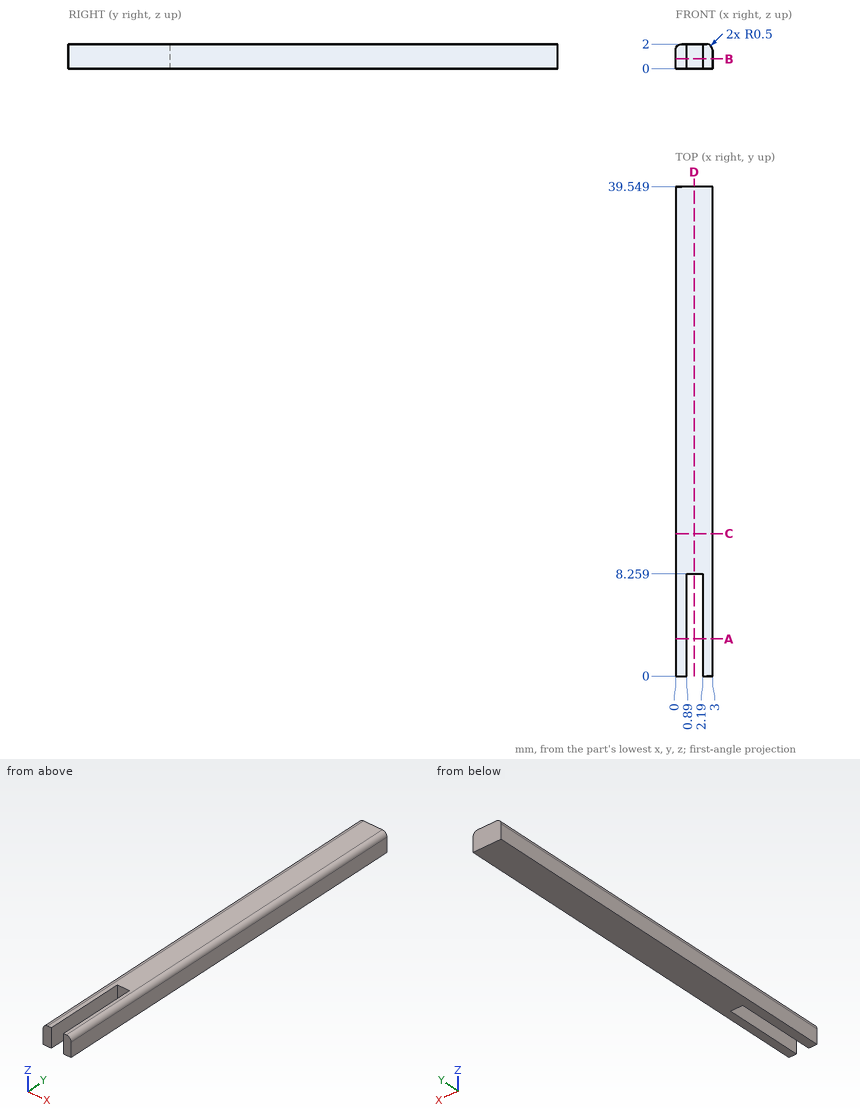
Check sheet for the drawn part. Datum: minimum x, y, z corner. Units: mm. Give positions to 0.01 mm unless a question says otherwise; leave off trailing zeros. Order: outer loops, then holes, each group sorted by start corner. A loop starts at its lowest first (then second) coordinate and runs counter-clockwise, first axis right, second up. Notation, with made-up numbers: (1, 65) - (17, 65) arc R24 ccw to (17, 83) - close; hole circle Ø2 at (66, 56). An arc over 180 degrees is marked (long way). Answer as a JSON object with one key per item and string values.
(1) Cross-section at A-A (y = 3). Record the cut outline in (x, z).
Report:
{"outline": "(0, 0) - (0.89, 0) - (0.89, 2) - (0.5, 2) arc R0.5 ccw to (0, 1.5) - close; (2.19, 0) - (3, 0) - (3, 1.5) arc R0.5 ccw to (2.5, 2) - (2.19, 2) - close"}
(2) Material ranges on line 1 (X direction, y = 7, z = 0.6); line 2 (Y direction, x = 1.8, z = 1.4); line 3 (Z direction, x = 2.55, y = 21.5), recorded low to high.
Report:
{"line 1": "0 to 0.89, 2.19 to 3", "line 2": "8.26 to 39.55", "line 3": "0 to 2"}
(3) Cross-section at B-B (z = 0.8). Record the cut outline in (x, y).
Report:
{"outline": "(0, 0) - (0.89, 0) - (0.89, 8.26) - (2.19, 8.26) - (2.19, 0) - (3, 0) - (3, 39.55) - (0, 39.55) - close"}
(4) Cross-section at D-D (x = 1.5). Record the cut outline in (y, z).
Report:
{"outline": "(8.26, 0) - (39.55, 0) - (39.55, 2) - (8.26, 2) - close"}
(5) Depth check by flat-ended pin: pin 1 Ø0.6 at (y, z) = (3.5, 1) entering from -X. Enter the tip coordinate at first touch or a pass-through.
Report:
{"pin 1": "x = 0"}
(6) Cross-section at C-C (y = 11.5). Record the cut outline in (x, z).
Report:
{"outline": "(0, 0) - (3, 0) - (3, 1.5) arc R0.5 ccw to (2.5, 2) - (0.5, 2) arc R0.5 ccw to (0, 1.5) - close"}
